Geometry: final body of the model. Coordinates: model frame, mm. Face numbers are marked on the shaded views. A direction names the side the tool comes from. Give positions to 0.01 mm unless a question says otherwise; leave off trailing zeros. Write each loop counter-clockwise with the first axis right and the second up, starting at its lowest first coordinate (ties: lowest second). Pieces come first, ordered by that corner, then holes. Notation, with made-up numbers: (34, -11) -> (92, -11) arc R30 cw to (92, 20) -> close; hole circle Ø4 at (-3.75, -26). An arc over 180 degrees is marked (long way). Answer as a JSON object with one key per item and string values. Group by question number.
(1) Set-up query: the marked faces 1, 2 and 3. Return all of +Z, -Z, +X, -X, +Y, -Y with unobstructed straight access to the full face (end or side cutting, diameter ignored); none if empty.
(2) Draft query along X for the marked faces 4, 5, 6 and 7. Return one class per face: +X half, -X half, draft (parallel to the pull), parting line (faces both ways), or undercut.
(3) Section query D-D on y = 28.5. Output: boundary loops of the cut face in (x, z).
(4) Section query A-A on y = 60. Output: boundary loops of the cut face in (x, z), plus the area to 3 significant figures.
(5) Contact query for flat-ended pins moving along their axis: pin 1 Ø15 at (y, z) = (36, 37.5) entering from +X; pin 2 Ø5 at (y, z) = (35, 39) entering from +X; pin 3 Ø6.5 at (x, z) = (-14.5, 25.5) entering from +Y; pin 4 Ø10 at (y, z) = (10.5, 35.5) entering from -X. Output: stop coordinate, or through.
(6) Section query B-B on z = 33.5. Output: boundary loops of the cut face in (x, y).
(7) Material intervals for probe 1 along Z at (x, y) = (15.5, 35); probe 2 along X at (y, z) = (42.5, 5.5); probe 3 along Z at (x, y) = (3, 36), sorted ascending.
(8) Section query C-C on x = -24. Output: boundary loops of the cut face in (y, z), plus the area to 3 significant figures.
from build123d import *

# Parameters (mm, degrees)
F0_W     = 70
F0_H     = 70
F1_DEPTH = 4
F2_W     = 8
F2_H     = 30
F3_DEPTH = 50
F4_R     = 14.99999
F7_D     = 6.5
F7_DEPTH = 15
F7_TIP   = 1.9527970118
F8_D     = 4
F8_DEPTH = 15
F8_TIP   = 1.2017212381


# Not quite as in the source:
# - a fillet or chamfer is up to 0.001 mm smaller than in the source, because OpenCascade refuses the exact size


with BuildPart() as f1:
    # F0 (on Top) → F1 (new body)
    with BuildSketch(Plane.XY):
        with Locations((1.0378739359, 35)):
            Rectangle(F0_W, F0_H)
    extrude(amount=F1_DEPTH)

    # F2 (on face) → F3 (join)
    with BuildSketch(Plane.XY.offset(4)):
        with Locations((-13.9621260641, 35)):
            Rectangle(F2_W, F2_H)
        with Locations((16.0378739359, 35)):
            Rectangle(F2_W, F2_H)
    extrude(amount=F3_DEPTH)

    # F4 (radius 15 in the source; OpenCascade refuses exactly that, so slightly less here)
    f4_edges = [f1.edges().sort_by_distance(p)[0] for p in [
        (-13.962126, 20, 54),
        (-13.962126, 50, 54),
        (16.037874, 20, 54),
        (16.037874, 50, 54),
    ]]
    fillet(f4_edges, radius=F4_R)

    # F7
    with Locations(Plane.YZ.offset(20.0378739359)):
        with Locations((35, 39)):
            Hole(F7_D / 2, depth=F7_DEPTH)
            with Locations((0, 0, -(F7_DEPTH + F7_TIP / 2))):  # 118° drill point
                Cone(0, F7_D / 2, F7_TIP, mode=Mode.SUBTRACT)

    # F8
    with Locations(Plane.XY.offset(4)):
        with Locations((-23.9621260641, 10), (26.0378739359, 10), (26.0378739359, 60), (-23.9621260641, 60)):
            Hole(F8_D / 2, depth=F8_DEPTH)
            with Locations((0, 0, -(F8_DEPTH + F8_TIP / 2))):  # 118° drill point
                Cone(0, F8_D / 2, F8_TIP, mode=Mode.SUBTRACT)


solid = f1.part
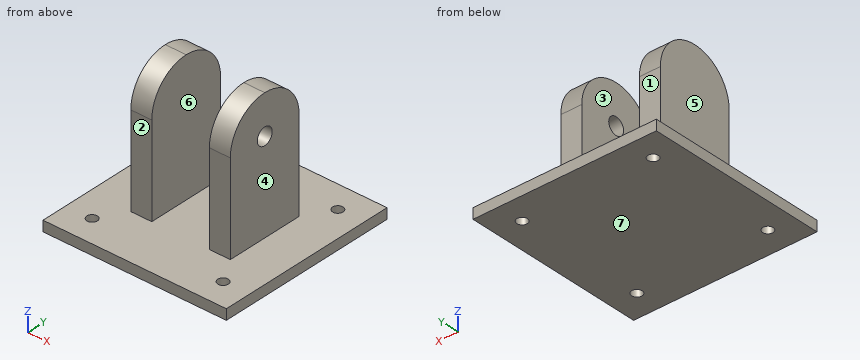
Answer list:
{
 "1": {"face 1": "+Z, +X, -X, +Y", "face 2": "+Z, +X, -X, -Y", "face 3": "+Z, +Y, -Y"},
 "2": {"face 4": "+X half", "face 5": "-X half", "face 6": "undercut", "face 7": "draft"},
 "3": {"outline": "(-33.96, 0) -> (36.04, 0) -> (36.04, 4) -> (20.04, 4) -> (20.04, 52.52) -> (12.04, 52.52) -> (12.04, 4) -> (-9.96, 4) -> (-9.96, 52.52) -> (-17.96, 52.52) -> (-17.96, 4) -> (-33.96, 4) -> close"},
 "4": {"outline": "(-33.96, 0) -> (-25.96, 0) -> (-25.96, 4) -> (-33.96, 4) -> close; (-21.96, 0) -> (24.04, 0) -> (24.04, 4) -> (-21.96, 4) -> close; (28.04, 0) -> (36.04, 0) -> (36.04, 4) -> (28.04, 4) -> close", "area": "248 mm2"},
 "5": {"pin 1": "x = 20.04", "pin 2": "x = -9.96", "pin 3": "y = 50", "pin 4": "through"},
 "6": {"outline": "(-17.96, 20) -> (-9.96, 20) -> (-9.96, 50) -> (-17.96, 50) -> close; (12.04, 20) -> (20.04, 20) -> (20.04, 50) -> (12.04, 50) -> close"},
 "7": {"probe 1": "0 to 35.75, 42.25 to 54", "probe 2": "-17.96 to -9.96, 12.04 to 20.04", "probe 3": "0 to 4"},
 "8": {"outline": "(0, 0) -> (8, 0) -> (8, 4) -> (0, 4) -> close; (12, 0) -> (58, 0) -> (58, 4) -> (12, 4) -> close; (62, 0) -> (70, 0) -> (70, 4) -> (62, 4) -> close", "area": "248 mm2"}
}
